from build123d import *

# Parameters (mm, degrees)
SKETCH1_R             = 3
SKETCH1_R_2           = 1.5
BOSS_EXTRUDE1_DEPTH   = 0.2
BOSS_EXTRUDE1_2_DEPTH = 0.2
BOSS_EXTRUDE1_3_DEPTH = 0.2
BOSS_EXTRUDE1_4_DEPTH = 0.2
SKETCH1_14_R          = 3.5
BOSS_EXTRUDE2_DEPTH   = 1
SKETCH1_17_R          = 3.5
SKETCH1_17_R_2        = 3
BOSS_EXTRUDE4_DEPTH   = 5


with BuildPart() as part:
    # Sketch1 → Boss-Extrude1 (new body)
    with BuildSketch(Plane(origin=(0, 0, 0), x_dir=(1, 0, 0), z_dir=(0, 1, 0))):
        with Locations(Location((347.273609729, 3.609230825, 0), (0, 0, 270))):
            Circle(SKETCH1_R)
        with Locations(Location((347.273609729, 3.609230825, 0), (0, 0, 270))):
            Circle(SKETCH1_R_2, mode=Mode.SUBTRACT)
    extrude(amount=BOSS_EXTRUDE1_DEPTH)



with BuildPart() as body_2:
    # Sketch1 → Boss-Extrude1 2 (new body)
    with BuildSketch(Plane(origin=(0, 0, 0), x_dir=(1, 0, 0), z_dir=(0, 1, 0))):
        with Locations(Location((410.793152563, -106.417182487, 0), (0, 0, 270))):
            Circle(SKETCH1_R)
        with Locations(Location((410.793152563, -106.417182487, 0), (0, 0, 270))):
            Circle(SKETCH1_R_2, mode=Mode.SUBTRACT)
    extrude(amount=BOSS_EXTRUDE1_2_DEPTH)


with BuildPart() as body_3:
    # Sketch1 → Boss-Extrude1 3 (new body)
    with BuildSketch(Plane(origin=(0, 0, 0), x_dir=(1, 0, 0), z_dir=(0, 1, 0))):
        with Locations(Location((283.758521159, -106.426112565, 0), (0, 0, 270))):
            Circle(SKETCH1_R)
        with Locations(Location((283.758521159, -106.426112565, 0), (0, 0, 270))):
            Circle(SKETCH1_R_2, mode=Mode.SUBTRACT)
    extrude(amount=BOSS_EXTRUDE1_3_DEPTH)


with BuildPart() as body_4:
    # Sketch1 → Boss-Extrude1 4 (new body)
    with BuildSketch(Plane(origin=(0, 0, 0), x_dir=(1, 0, 0), z_dir=(0, 1, 0))):
        Polygon((231.981171214, -138.914415757), (229.712705007, -134.986323544), (344.980692969, 64.663360453), (349.516789508, 64.663360453), (464.784783451, -134.986661544), (462.517056767, -138.914415757), align=None)
        Polygon((243.304219773, -116.484791866), (254.809280576, -136.408896139), (442.602090749, -136.409305398), (452.699916625, -118.984688015), (358.778179035, 43.666038066), (335.767496284, 43.666038066), align=None, mode=Mode.SUBTRACT)
    extrude(amount=BOSS_EXTRUDE1_4_DEPTH)

    # Sketch1_14 → Boss-Extrude2 (add)
    with BuildSketch(Plane(origin=(0, 0, 0), x_dir=(1, 0, 0), z_dir=(0, 1, 0))):
        Polygon((243.304219773, -116.484791866), (254.809280576, -136.408896139), (442.602090749, -136.409305398), (452.699916625, -118.984688015), (358.778179035, 43.666038066), (335.767496284, 43.666038066), align=None)
        with Locations(Location((347.273609729, 3.609230825, 0), (0, 0, 270))):
            Circle(SKETCH1_14_R, mode=Mode.SUBTRACT)
        with Locations(Location((410.793152563, -106.417182487, 0), (0, 0, 270))):
            Circle(SKETCH1_14_R, mode=Mode.SUBTRACT)
        with Locations(Location((283.758521159, -106.426112565, 0), (0, 0, 270))):
            Circle(SKETCH1_14_R, mode=Mode.SUBTRACT)
    extrude(amount=BOSS_EXTRUDE2_DEPTH)


with BuildPart() as part_1:
    add(part.part)

    add(body_2.part)  # Boss-Extrude4 merges body 2

    add(body_3.part)  # Boss-Extrude4 merges body 3

    add(body_4.part)  # Boss-Extrude4 merges body 4
    # Sketch1_17 → Boss-Extrude4 (add)
    # profile 1 of 3: a face of its own
    with BuildSketch(Plane(origin=(0, 0, 0), x_dir=(1, 0, 0), z_dir=(0, 1, 0))):
        with Locations(Location((283.758521159, -106.426112565, 0), (0, 0, 270))):
            Circle(SKETCH1_17_R)
        with Locations(Location((283.758521159, -106.426112565, 0), (0, 0, 270))):
            Circle(SKETCH1_17_R_2, mode=Mode.SUBTRACT)
    # profile 2 of 3: a face of its own
    with BuildSketch(Plane(origin=(0, 0, 0), x_dir=(1, 0, 0), z_dir=(0, 1, 0))):
        with Locations(Location((410.793152563, -106.417182487, 0), (0, 0, 270))):
            Circle(SKETCH1_17_R)
        with Locations(Location((410.793152563, -106.417182487, 0), (0, 0, 270))):
            Circle(SKETCH1_17_R_2, mode=Mode.SUBTRACT)
    # profile 3 of 3: a face of its own
    with BuildSketch(Plane(origin=(0, 0, 0), x_dir=(1, 0, 0), z_dir=(0, 1, 0))):
        with Locations(Location((347.273609729, 3.609230825, 0), (0, 0, 270))):
            Circle(SKETCH1_17_R)
        with Locations(Location((347.273609729, 3.609230825, 0), (0, 0, 270))):
            Circle(SKETCH1_17_R_2, mode=Mode.SUBTRACT)
    extrude(amount=BOSS_EXTRUDE4_DEPTH)


solid = part_1.part
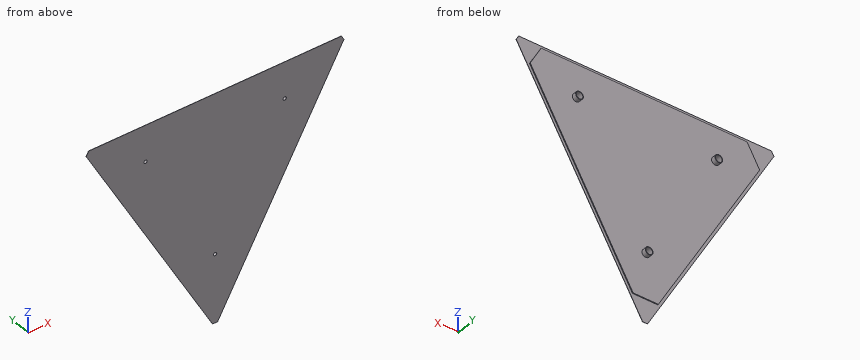
Verification items for the finished model (mm, model axes). Coordinates: 2 decimals unless noted, no trailing zeros. Order: outer loops, then holes, each group sorted by start corner. A loop starts at its lowest first (then second) coordinate and runs counter-clockwise, first axis right, second up.
1. Scan lines: line 1 (Y direction, x = 375, z = 25.5); line 2 (Z direction, x = 349.5, y = 1.95); line 3 (Z direction, x = 341.5, y = 0.9). Record each from-to range of solid material in increasing order.
Results found:
line 1: y = 0 to 1
line 2: z = -6.31 to -5.62, -1.6 to -0.91
line 3: z = -43.67 to 136.41
2. Sectioned sample at C-C, the plane z = 83.5. Record the cut outline in (x, y).
Results found:
outline: (259.44, 0) - (435.06, 0) - (435.06, 0.2) - (432.21, 0.2) - (432.21, 1) - (262.35, 1) - (262.35, 0.2) - (259.44, 0.2) - close
3. Go/stop test with flat-tipped pins: pin 1 Ø5 at (x, z) = (284, 106.5) entering from +Y; pin 2 Ø0.6 at (x, y) = (317, 1) entering from +Z; pin 3 Ø6 at (x, z) = (324.5, -23) entering from +Y. Record where each tip stops, or that it passes through.
Results found:
pin 1: stops at y = 0.2
pin 2: stops at z = 136.41
pin 3: stops at y = 1
4. Sectioned sample at B-B, the plane x = 437.5. Record the cut outline in (y, z).
Results found:
outline: (0, 87.73) - (0.2, 87.73) - (0.2, 92.66) - (1, 92.66) - (1, 136.41) - (0.2, 136.41) - (0.2, 138.91) - (0, 138.91) - close
5. Sectioned sample at A-A, the plane y = 4.1. Record the cut outline in (x, z).
Results found:
outline: circle Ø7 at (283.76, 106.43); circle Ø7 at (347.27, -3.61); circle Ø7 at (410.79, 106.42); hole circle Ø6 at (283.76, 106.43); hole circle Ø6 at (347.27, -3.61); hole circle Ø6 at (410.79, 106.42)
